```python
from build123d import *

# Parameters (mm, degrees)
F0_W     = 355.6
F0_H     = 355.6
F1_DEPTH = 38.1
F2_DEPTH = 76.2


with BuildPart() as f1:
    # F0 (on Front) → F1 (new body)
    with BuildSketch(Plane.XZ):
        with Locations((1122.902123, -4376.915325)):
            Rectangle(F0_W, F0_H)
        Polygon((945.102123, -3894.315325), (945.102123, -4199.115325), (1300.702123, -4199.115325), (1300.702123, -4554.715325), (1605.502123, -4554.715325), (1605.502123, -4199.115325), (1961.102123, -4199.115325), (1961.102123, -3894.315325), (1605.502123, -3894.315325), (1605.502123, -3538.715325), (1300.702123, -3538.715325), (1300.702123, -3894.315325), align=None)
        with Locations((1783.302123, -4376.915325)):
            Rectangle(F0_W, F0_H)
        with Locations((1783.302123, -3716.515325)):
            Rectangle(F0_W, F0_H)
        with Locations((1122.902123, -3716.515325)):
            Rectangle(F0_W, F0_H)
    extrude(amount=F1_DEPTH)

    # F0 (on Front) → F2 (join)
    with BuildSketch(Plane.XZ):
        with Locations((1783.302123, -3716.515325)):
            Rectangle(F0_W, F0_H)
        with Locations((1783.302123, -4376.915325)):
            Rectangle(F0_W, F0_H)
        with Locations((1122.902123, -4376.915325)):
            Rectangle(F0_W, F0_H)
        with Locations((1122.902123, -3716.515325)):
            Rectangle(F0_W, F0_H)
    extrude(amount=F2_DEPTH)


solid = f1.part
```
Source: CAD feature listing. Evaluate the final solid. Frame: model axes, mm. A direction names the side the tool comes from. Round coordinates to 2 decimals unless told otherwise and drop trailing zeros. Order: outer loops, then holes, each group sorted by start corner. A loop starts at its lowest first (then second) coordinate and runs counter-clockwise, first axis right, second up. Notation, with made-up numbers: (-3, 70) -> (20, 70) arc R30 cw to (20, 100) -> close; hole circle Ø8 at (-4, -2.5). An arc over 180 degrees is marked (long way). One line per item, written item: value. Start each with the question number.
Q1. Material intervals for probe 1 along X at (y, z) = (-65.5, -3719); probe 2 along Z at (x, y) = (1040, -59); probe 3 along Y at (x, z) = (1217.5, -4028), sorted ascending.
Q2. Section query B-B (z = -3665). Return the cut outline in (x, y).
Q3. Pin query (flat end, axial travel): pin 1 (1 mm diameter, centred on x = 1611.5, z = -3975.5, fed in from -Y). Return the tip coordinate at first contact, or that it passes through.
Q4. Draft query along X for faces 1 (the flat face through (1120, -76.2, -4374)), 2 (the flat face through (945.102, -37.6, -4039.6)), 3 (the flat face through (1300.702, -57, -4379)). Return one class per face: pulls with the +X half, pulls with the -X half, needs draft (parallel to the pull), parting line crosses it, or undercut.
Q5. Section query C-C (x = 1723.5). Return the cut outline in (y, z).
Q6. Section query D-D (x = 1376). Return the cut outline in (y, z).
Q7. Section query A-A (y = -63). Return the cut outline in (x, z), plus the area to 3 significant figures.
Q8. Access query for faces 4 (the flat face through (1300.702, -57, -3719)), 5 (the flat face through (1446, 0, -4040)), 6 (the flat face through (1781, -57, -3894.315)). Directions: +Z, -Z, +X, -X, +Y, -Y. A direction counts if a zero-diameter tool reaches every point of the face in a straight line with its end or side. Return the directions, or none.
Findings below:
1. probe 1: 945.1 to 1300.7, 1605.5 to 1961.1
1. probe 2: -4554.72 to -4199.12, -3894.32 to -3538.72
1. probe 3: -38.1 to 0
2. outline: (945.1, -76.2) -> (1300.7, -76.2) -> (1300.7, -38.1) -> (1605.5, -38.1) -> (1605.5, -76.2) -> (1961.1, -76.2) -> (1961.1, 0) -> (945.1, 0) -> close
3. pin 1: y = -38.1
4. face 1: needs draft
4. face 2: pulls with the -X half
4. face 3: undercut
5. outline: (-76.2, -4554.72) -> (0, -4554.72) -> (0, -3538.72) -> (-76.2, -3538.72) -> (-76.2, -3894.32) -> (-38.1, -3894.32) -> (-38.1, -4199.12) -> (-76.2, -4199.12) -> close
6. outline: (-38.1, -4554.72) -> (0, -4554.72) -> (0, -3538.72) -> (-38.1, -3538.72) -> close
7. outline: (945.1, -4554.72) -> (1300.7, -4554.72) -> (1300.7, -4199.12) -> (945.1, -4199.12) -> close; (945.1, -3894.32) -> (1300.7, -3894.32) -> (1300.7, -3538.72) -> (945.1, -3538.72) -> close; (1605.5, -4554.72) -> (1961.1, -4554.72) -> (1961.1, -4199.12) -> (1605.5, -4199.12) -> close; (1605.5, -3894.32) -> (1961.1, -3894.32) -> (1961.1, -3538.72) -> (1605.5, -3538.72) -> close
7. area: 506,000 mm²
8. face 4: +Z, -Z, -Y
8. face 5: +Z, -Z, +X, -X, +Y
8. face 6: +X, -X, -Y
